Autodesk Inventor part; units mm, degrees
ref_plane "YZ Plane" through (0, 0, 0) normal (1, 0, 0) x (0, 1, 0)
ref_plane "XZ Plane" through (0, 0, 0) normal (0, 1, 0) x (-1, 0, 0)
ref_plane "XY Plane" through (0, 0, 0) normal (0, 0, 1) x (1, 0, 0)
sketch "草圖1" plane through (0, 0, 0) normal (0, 1, 0) x (-1, 0, 0)
  line L0 (42, 0) -> (-42, 0)
  line L1 (0, -77.6) -> (0, 87.6)
  line L2 (-30, 0) -> (-30, 64)
  line L3 (-30, 64) -> (30, 64)
  line L4 (30, 64) -> (30, 0)
  line L5 (21, 0) -> (21, -7.5)
  line L6 (21, -7.5) -> (0, -7.5)
  line L7 (0, -7.5) -> (24, -7.5)
  line L8 (24, -7.5) -> (24, -17.5)
  line L9 (24, -17.5) -> (0, -17.5)
  line L10 (0, -17.5) -> (0, -7.5)
  line L11 (0, -17.5) -> (21, -17.5)
  line L12 (21, -17.5) -> (21, -42.5)
  line L13 (21, -42.5) -> (0, -42.5)
  line L14 (0, -42.5) -> (0, -17.5)
  line L15 (0, -42.5) -> (24, -42.5)
  line L16 (24, -42.5) -> (24, -52.5)
  line L17 (24, -52.5) -> (0, -52.5)
  line L18 (0, -52.5) -> (0, -42.5)
  line L19 (0, -52.5) -> (21, -52.5)
  line L20 (21, -52.5) -> (21, -54)
  line L21 (21, -54) -> (0, -54)
  line L22 (0, -54) -> (0, -52.5)
  line L23 (-21, 0) -> (-21, -7.5)
  line L24 (-21, -7.5) -> (0, -7.5)
  line L25 (0, -7.5) -> (-24, -7.5)
  line L26 (-24, -7.5) -> (-24, -17.5)
  line L27 (-24, -17.5) -> (0, -17.5)
  line L28 (0, -17.5) -> (-21, -17.5)
  line L29 (-21, -17.5) -> (-21, -42.5)
  line L30 (-21, -42.5) -> (0, -42.5)
  line L31 (0, -42.5) -> (-24, -42.5)
  line L32 (-24, -42.5) -> (-24, -52.5)
  line L33 (-24, -52.5) -> (0, -52.5)
  line L34 (0, -52.5) -> (-21, -52.5)
  line L35 (-21, -52.5) -> (-21, -54)
  line L36 (-21, -54) -> (0, -54)
  line L37 (30, 0) -> (21, 0)
  line L38 (-21, 0) -> (-30, 0)
  point P0 (0, 0)
  dimension "d0" = 60
  dimension "d1" = 64
  dimension "d2" = 30
  dimension "d3" = 9
  dimension "d4" = 7.5
  dimension "d5" = 10
  dimension "d6" = 3
  dimension "d7" = 25
  dimension "d8" = 10
  dimension "d9" = 3
  dimension "d10" = 9
  dimension "d11" = 1.5
extrude "擠出1" add sketch "草圖1" along normal mid plane 3
sketch "草圖2" plane through (0, 1.5, 0) normal (0, 1, 0) x (1, 0, 0)
  line L0 (-21, 52.5) -> (-21, 54)
  line L1 (-21, 54) -> (21, 54)
  line L2 (21, 54) -> (21, 52.5)
  line L3 (21, 52.5) -> (24, 52.5)
  line L4 (24, 52.5) -> (24, 42.5)
  line L5 (24, 42.5) -> (21, 42.5)
  line L6 (21, 42.5) -> (21, 17.5)
  line L7 (21, 17.5) -> (24, 17.5)
  line L8 (24, 17.5) -> (24, 7.5)
  line L9 (24, 7.5) -> (21, 7.5)
  line L10 (21, 7.5) -> (21, 0)
  line L11 (21, 0) -> (30, 0)
  line L12 (30, 0) -> (30, -64)
  line L13 (30, -64) -> (-30, -64)
  line L14 (-30, -64) -> (-30, 0)
  line L15 (-30, 0) -> (-21, 0)
  line L16 (-21, 0) -> (-21, 7.5)
  line L17 (-21, 7.5) -> (-24, 7.5)
  line L18 (-24, 7.5) -> (-24, 17.5)
  line L19 (-24, 17.5) -> (-21, 17.5)
  line L20 (-21, 17.5) -> (-21, 42.5)
  line L21 (-21, 42.5) -> (-24, 42.5)
  line L22 (-24, 42.5) -> (-24, 52.5)
  line L23 (-24, 52.5) -> (-21, 52.5)
  line L24 (-21, 28.5) -> (-17, 28.5)
  line L25 (-17, 28.5) -> (-17, 31.5)
  line L26 (-17, 31.5) -> (-21, 31.5)
  line L27 (-21, 31.5) -> (-21, 28.5)
  line L28 (-17, 26) -> (-14.5, 26)
  line L29 (-14.5, 26) -> (-14.5, 34)
  line L30 (-14.5, 34) -> (-17, 34)
  line L31 (-17, 34) -> (-17, 26)
  line L32 (-14.5, 28.5) -> (-13, 28.5)
  line L33 (-13, 28.5) -> (-13, 31.5)
  line L34 (-13, 31.5) -> (-14.5, 31.5)
  line L35 (-14.5, 31.5) -> (-14.5, 28.5)
  line L36 (0, 0) -> (0, 17.5)
  line L37 (21, 28.5) -> (17, 28.5)
  line L38 (17, 28.5) -> (17, 31.5)
  line L39 (17, 31.5) -> (21, 31.5)
  line L40 (17, 26) -> (14.5, 26)
  line L41 (14.5, 26) -> (14.5, 34)
  line L42 (14.5, 34) -> (17, 34)
  line L43 (17, 34) -> (17, 26)
  line L44 (14.5, 28.5) -> (13, 28.5)
  line L45 (13, 28.5) -> (13, 31.5)
  line L46 (13, 31.5) -> (14.5, 31.5)
  line L47 (14.5, 31.5) -> (14.5, 28.5)
  line L48 (21, 28.5) -> (21, 31.5)
  line L49 (21, 42.5) -> (21, 17.5)
  dimension "d14" = 3
  dimension "d15" = 11
  dimension "d16" = 4
  dimension "d17" = 2.5
  dimension "d18" = 1.5
  dimension "d19" = 2.5
  dimension "d20" = 2.5
extrude "擠出2" cut sketch "草圖2" against normal blind 10 contours L26 L25 L24 L20 | L31 L30 L29 L28 L25 | L6 L37 L38 L39 | L38 L43 L40 L41 L42 | L34 L33 L32 L29 | L41 L44 L45 L46
sketch "草圖3" plane through (0, 1.5, 0) normal (0, 1, 0) x (1, 0, 0)
  line L0 (-21, 28.5) -> (-17, 28.5)
  line L1 (-17, 28.5) -> (-17, 26)
  line L2 (-17, 26) -> (-14.5, 26)
  line L3 (-14.5, 26) -> (-14.5, 28.5)
  line L4 (-14.5, 28.5) -> (-13, 28.5)
  line L5 (-13, 28.5) -> (-13, 31.5)
  line L6 (-13, 31.5) -> (-14.5, 31.5)
  line L7 (-14.5, 31.5) -> (-14.5, 34)
  line L8 (-14.5, 34) -> (-17, 34)
  line L9 (-17, 34) -> (-17, 31.5)
  line L10 (-17, 31.5) -> (-21, 31.5)
  line L11 (-21, 31.5) -> (-21, 42.5)
  line L12 (-21, 42.5) -> (-24, 42.5)
  line L13 (-24, 42.5) -> (-24, 52.5)
  line L14 (-24, 52.5) -> (-21, 52.5)
  line L15 (-21, 52.5) -> (-21, 54)
  line L16 (-21, 54) -> (21, 54)
  line L17 (21, 54) -> (21, 52.5)
  line L18 (21, 52.5) -> (24, 52.5)
  line L19 (24, 52.5) -> (24, 42.5)
  line L20 (24, 42.5) -> (21, 42.5)
  line L21 (21, 42.5) -> (21, 31.5)
  line L22 (21, 31.5) -> (17, 31.5)
  line L23 (17, 31.5) -> (17, 34)
  line L24 (17, 34) -> (14.5, 34)
  line L25 (14.5, 34) -> (14.5, 31.5)
  line L26 (14.5, 31.5) -> (13, 31.5)
  line L27 (13, 31.5) -> (13, 28.5)
  line L28 (13, 28.5) -> (14.5, 28.5)
  line L29 (14.5, 28.5) -> (14.5, 26)
  line L30 (14.5, 26) -> (17, 26)
  line L31 (17, 26) -> (17, 28.5)
  line L32 (17, 28.5) -> (21, 28.5)
  line L33 (21, 28.5) -> (21, 17.5)
  line L34 (21, 17.5) -> (24, 17.5)
  line L35 (24, 17.5) -> (24, 7.5)
  line L36 (24, 7.5) -> (21, 7.5)
  line L37 (21, 7.5) -> (21, 0)
  line L38 (21, 0) -> (30, 0)
  line L39 (30, 0) -> (30, -64)
  line L40 (30, -64) -> (-30, -64)
  line L41 (-30, -64) -> (-30, 0)
  line L42 (-30, 0) -> (-21, 0)
  line L43 (-21, 0) -> (-21, 7.5)
  line L44 (-21, 7.5) -> (-24, 7.5)
  line L45 (-24, 7.5) -> (-24, 17.5)
  line L46 (-24, 17.5) -> (-21, 17.5)
  line L47 (-21, 17.5) -> (-21, 28.5)
  line L48 (-30, 0) -> (-21, 0)
  line L49 (-30, 0) -> (-27, 0)
  line L50 (-27, 0) -> (-27, -11.7)
  line L51 (-27, -11.7) -> (-24.2, -11.7)
  line L52 (-24.2, -11.7) -> (-24.2, -16.8)
  circle A0 centre (-27, -11.7) radius 1.5
  circle A1 centre (-24.2, -16.8) radius 1.5
  line L53 (-27, -11.7) -> (-27, -21.7)
  circle A2 centre (-27, -21.7) radius 0.75
  line L54 (-27, -21.7) -> (-27, -34.7)
  circle A3 centre (-27, -34.7) radius 1.5
  line L55 (-27, -34.7) -> (-27, -48.7)
  circle A4 centre (-27, -48.7) radius 0.75
  line L56 (-27, -48.7) -> (-27, -44.7)
  line L57 (-27, -44.7) -> (-24.2, -44.7)
  circle A5 centre (-24.2, -44.7) radius 1.5
  line L58 (30, -64) -> (-30, -64)
  line L59 (0, -64) -> (0, 30)
  circle A6 centre (27, -11.7) radius 1.5
  circle A7 centre (27, -34.7) radius 1.5
  circle A8 centre (25.7, -60) radius 1.5
  circle A9 centre (16.5, -5.4) radius 1.3
  circle A10 centre (-2.3, -5.4) radius 1.3
  circle A11 centre (-5.7, -35.26) radius 0.75
  line L60 (-13, 28.5) -> (-13, 31.5)
  line L61 (-13, 30) -> (13, 30)
  line L62 (13, 31.5) -> (13, 28.5)
  circle A12 centre (0, 30) radius 1.5
  circle A13 centre (0, 30) radius 3.6
  circle A14 centre (0, 19) radius 0.75
  circle A15 centre (-6.7, 30) radius 0.75
  circle A16 centre (6.7, 30) radius 0.75
  circle A17 centre (0, 41) radius 0.75
  circle A18 centre (-2.3, 50.5) radius 1.3
  circle A19 centre (16.5, 50.5) radius 1.3
  circle A20 centre (-8.7, 48.75) radius 1.5
  point P0 (0, 0)
  dimension "d23" = 3
  dimension "d24" = 11.7
  dimension "d25" = 2.8
  dimension "d26" = 5.1
  dimension "d27" = 3
  dimension "d28" = 3
  dimension "d29" = 10
  dimension "d30" = 1.5
  dimension "d31" = 13
  dimension "d32" = 3
  dimension "d33" = 14
  dimension "d34" = 1.5
  dimension "d35" = 4
  dimension "d36" = 3
  dimension "d37" = 94
  dimension "d38" = 4.3
  dimension "d39" = 4
  dimension "d40" = 3
  dimension "d41" = 2.6
  dimension "d42" = 5.4
  dimension "d43" = 13.5
  dimension "d44" = 2.6
  dimension "d46" = 5.4
  dimension "d47" = 28.74
  dimension "d48" = 35.7
  dimension "d49" = 1.5
  dimension "d50" = 3
  dimension "d51" = 7.2
  dimension "d52" = 6.7
  dimension "d53" = 11
  dimension "d54" = 1.5
  dimension "d55" = 1.5
  dimension "d56" = 18.8
  dimension "d58" = 2.6
  dimension "d60" = 2.6
  dimension "d63" = 3
extrude "擠出3" cut sketch "草圖3" against normal blind 10 contours A1 | A5 | A4 | A3 L55 L54 | L54 L55 A3 | A2 L54 L53 | L53 L54 A2 | A0 L51 L50 | L50 L53 A0 | A15 L61 | L61 A15 | L51 A0 L53 | A14 L59 | L59 A14 | A6 | A7 | A8 | A9 | A10 | A11
extrude "擠出4" cut sketch "草圖3" against normal blind 10 contours A13 L61 A12 | L61 A12 L59 A13 | A12 L61 | L61 L59 A12 | A13 L59 A12 L61 | L61 A12 L59 | A16 L61 | L61 A16 | A17
extrude "擠出5" cut sketch "草圖3" against normal blind 10 contours A18 | A19 | A20
properties part number "板子9"
Check sheet for the modelled part. Datum: model origin and axes. Units: mm. A direction names the side the tool comes from. Coordinates: 2 decimals unless noted, no trailing zeros. Loops run counter-clockwise (first coordinate to the right, second up) from the corner with the lowest first, then second, coordinate; pieces in that order, holes last. Notation, with made-up numbers: (11, 52.5) -> (52, 52.5) arc R27 cw to (52, 83.5) -> close; hole circle Ø2 at (-6.5, -29). An arc over 180 degrees is marked (long way). Answer in a Markdown table with one row per item.
1. Sectioned sample at A-A, the plane z = 16.8. Record the boundary of the cut face in (x, y), then the cut area to 3 significant figures.
Check values:
| item | result |
|---|---|
| outline | (-30, -1.5) -> (-25.7, -1.5) -> (-25.7, 1.5) -> (-30, 1.5) -> close; (-22.7, -1.5) -> (30, -1.5) -> (30, 1.5) -> (-22.7, 1.5) -> close |
| area | 171 mm2 |
2. Access from +Z, -Z, +X, -X, +Y, -Y to the whole of each face (thin tool, end or side, straight path). Record for faces 1 (the face through (-24, 0, -12)), 2 (the face through (16, 0, -34)), 3 (the face through (-21, 0, -37)), 4 (the face through (19, 0, -31.5)).
Check values:
| item | result |
|---|---|
| face 1 | -Z, -X, +Y, -Y |
| face 2 | +Y, -Y |
| face 3 | -X, +Y, -Y |
| face 4 | +X, +Y, -Y |
3. Release check for a two-part mould opening along X. For faces 5 (the face through (13, 0, -30)), 6 (the face through (-13, 0, -30)), 7 (the face through (25.5, 0.02, 11.63)), 8 (the face through (25, 0, 0)) record: released by +X, released by -X, zero draft, split by the parting line, or undercut.
Check values:
| item | result |
|---|---|
| face 5 | released by +X |
| face 6 | released by -X |
| face 7 | undercut |
| face 8 | zero draft |
4. Material ranges on line 1 along X through (y, z) = (-0.3, -50.5); line 2 along X through (y, z) = (0.95, -30); line 3 along Z through (x, y) = (-24.2, -0.4), recorded low to high. Write a range as [from, to].
Check values:
| item | result |
|---|---|
| line 1 | x = [-24, -3.6], [-1, 15.2], [17.8, 24] |
| line 2 | x = [-13, -7.45], [-5.95, -3.6], [3.6, 5.95], [7.45, 13] |
| line 3 | z = [0, 15.3], [18.3, 43.2], [46.2, 64] |
5. Go/stop test with flat-tipped pins: pin 1 (1.5 mm diameter, centred on y = -0.5, z = -38, fed in from +X); pin 2 (1 mm diameter, centred on y = 1, z = -17, fed in from -X); pin 3 (0.9 mm diameter, centred on x = 22, y = 0.5, fed in from -Z). Record where each tip stops, or that it passes through.
Check values:
| item | result |
|---|---|
| pin 1 | stops at x = 21 |
| pin 2 | stops at x = -24 |
| pin 3 | stops at z = -52.5 |
6. Sectioned sample at B-B, the plane y = 0.85. Give the number of separate pieces and of enclosed holes in the cut face, then the cut area to 3 significant figures.
Check values:
| item | result |
|---|---|
| separate pieces | 1 |
| enclosed holes | 20 |
| area | 6,020 mm2 |
